Input: part model. Units: mm. Frame: model coordinates. A direction names the side the tool comes from. Coordinates: 2 decimals unless noted, no trailing zeros. Write each loop counter-clockwise with the first axis right and the second up, starting at its lowest first coordinate (ties: lowest second). Pieces come first, ordered by that corner, then holes. Notation, with made-up numbers: (15, 40.25) - (24, 40.25) arc R18 cw to (24, 74.25) - close; hole circle Ø6 at (17, 85.5). An arc over 180 degrees is marked (long way). Put each result on its own line as item: value. Start each with the question number.
1. Line query: line 1 (X direction, y = -8.5, z = 6); line 2 (Y direction, x = 13.4, z = 0); line 3 (X direction, y = 0.5, z = 9.25). Output: solid intervals per line, ascending.
2. Access query for faces 1 (the cylindrical face through (-1.25, -2.38, 10.74)), 2 (the cylindrical face through (12.25, -2.38, -10.74)), 3 (the cylindrical face through (-0.246, 11.923, 3.755)). Directions: +Z, -Z, +X, -X, +Y, -Y. A direction counts if a zero-diameter tool reaches every point of the face in a straight line with its end or side. Return the directions, or none.
3. Cut plane B-B, the plane z = 0. Count the separate pieces of the cut face and the enclosed holes in it, and give its area (3 significant figures).
4. Pin query (flat end, axial travel): pin 1 (1.5 mm diameter, centred on y = 9, z = -3.5, fed in from -X); pin 2 (1 mm diameter, centred on y = -7.5, z = -7.5, fed in from +X). Return the tip coordinate at first contact, or that it passes through.
5. Cut plane A-A, the plane x = -4. Return loops of the section in (y, z).
6. Pull-direction query (Z, two-part tool) for faces 4 (the flat face through (16.1, 0, 0)), 5 (the cylindrical face through (14.028, -2.749, -8.447)), 6 (the cylindrical face through (15.75, -2.38, -10.74)); classes: released by +Z, released by -Z, zero draft, split by the parting line, or undercut.
Autodesk Inventor part; units mm, degrees
ref_plane "YZ Plane" through (0, 0, 0) normal (1, 0, 0) x (0, 1, 0)
ref_plane "XZ Plane" through (0, 0, 0) normal (0, 1, 0) x (-1, 0, 0)
ref_plane "XY Plane" through (0, 0, 0) normal (0, 0, 1) x (1, 0, 0)
sketch "Sketch1" plane through (0, 0, 0) normal (0, 0, 1) x (1, 0, 0)
  line L0 (0, 0) -> (0, 3)
  line L1 (0, 3) -> (12, 3)
  line L2 (12, 3) -> (12, 11)
  line L3 (12, 11) -> (12.5, 11)
  line L4 (12.5, 11) -> (12.5, 10)
  line L5 (12.5, 10) -> (15.5, 10)
  line L6 (15.5, 10) -> (15.5, 11)
  line L7 (15.5, 11) -> (16, 11)
  line L8 (16, 11) -> (16, 0)
  line L9 (16, 0) -> (0, 0)
  dimension "d0" = 3
  dimension "d1" = 12
  dimension "d2" = 0.5
  dimension "d3" = 10
  dimension "d4" = 0.5
  dimension "d5" = 1
  dimension "d6" = 3
revolve "Revolution1" add sketch "Sketch1" angle 360 about axis through (16, 0, 0) along (-1, 0, 0)
sketch "Sketch2" plane through (0, 0, 0) normal (0, 0, 1) x (1, 0, 0)
  line L0 (0, -3) -> (0, 3)
  line L1 (0, 0) -> (-2.5, 0)
  line L2 (-2.5, 0) -> (-2.5, 12.5)
  line L3 (-2.5, 12.5) -> (0, 12.5) construction
  line L4 (0, 12.5) -> (0, 0)
  line L5 (-1.25, 12.5) -> (-1.25, 11) construction
  line L6 (-1.25, 11) -> (-1.5981, 11)
  line L7 (-1.5981, 11) -> (-2, 12.5)
  line L8 (-0.9019, 11) -> (-0.5, 12.5)
  line L9 (-0.9019, 11) -> (-1.25, 11)
  line L10 (-2, 12.5) -> (-2.5, 12.5)
  line L11 (-0.5, 12.5) -> (0, 12.5)
  dimension "d8" = 12.5
  dimension "d9" = 2.5
  dimension "d10" = 1.5
  dimension "d11" = 15
  dimension "d12" = 0.75
revolve "Revolution2" add sketch "Sketch2" angle 360 about axis through (0, 0, 0) along (-1, 0, 0)
sketch "Sketch3" plane through (-2.5, 0, 0) normal (-1, 0, 0) x (0, 0, 1)
  circle A0 centre (0, 0) radius 12.5
  circle A1 centre (0, 0) radius 2
  dimension "d14" = 4
extrude "Extrusion1" add sketch "Sketch3" along normal blind 4 contours A1
sketch "Sketch4" plane through (16, 0, 0) normal (1, 0, 0) x (0, 0, -1)
  circle A0 centre (0, 0) radius 10.5
  circle A1 centre (0, 0) radius 10
  circle A2 centre (0, 0) radius 11
  circle A3 centre (0, 7) radius 2.5
  circle A4 centre (0, 0) radius 3 construction
  dimension "d17" = 7
  dimension "d18" = 5
  dimension "d19" = 6
extrude "Extrusion2" cut sketch "Sketch4" against normal through all contours A3
pattern_circular "Circular Pattern1" count 3 over 360 about axis through (6, 0, 0) along (1, 0, 0) of "Extrusion2"
sketch "Sketch5" plane through (16, 0, 0) normal (1, 0, 0) x (0, 0, -1)
  circle A0 centre (0, 0) radius 11
  circle A1 centre (0, 0) radius 2.5
  dimension "d25" = 5
extrude "Extrusion3" add sketch "Sketch5" along normal blind 0.1 contours A1
properties part number "PulleyMotor"
Report:
1. line 1: x = -2.5 to 0, 12 to 12.5, 15.5 to 16
1. line 2: y = -10 to 4.5, 9.5 to 10
1. line 3: x = -2.5 to 0, 12 to 16
2. face 1: none
2. face 2: +X
2. face 3: +X, -X
3. separate pieces: 3
3. enclosed holes: 0
3. area: 197 mm^2
4. pin 1: stops at x = -2.5
4. pin 2: stops at x = 16
5. outline: circle Ø4 at (0, 0)
6. face 4: zero draft
6. face 5: undercut
6. face 6: split by the parting line
